Source: three-view drawing plus pictorial views. Frame: mm from the lowest corner of the part. Give positions to 0.01 mm unless a question says otherwise; leave off trailing zeros. Return JSON: item names as keys, results as strings.
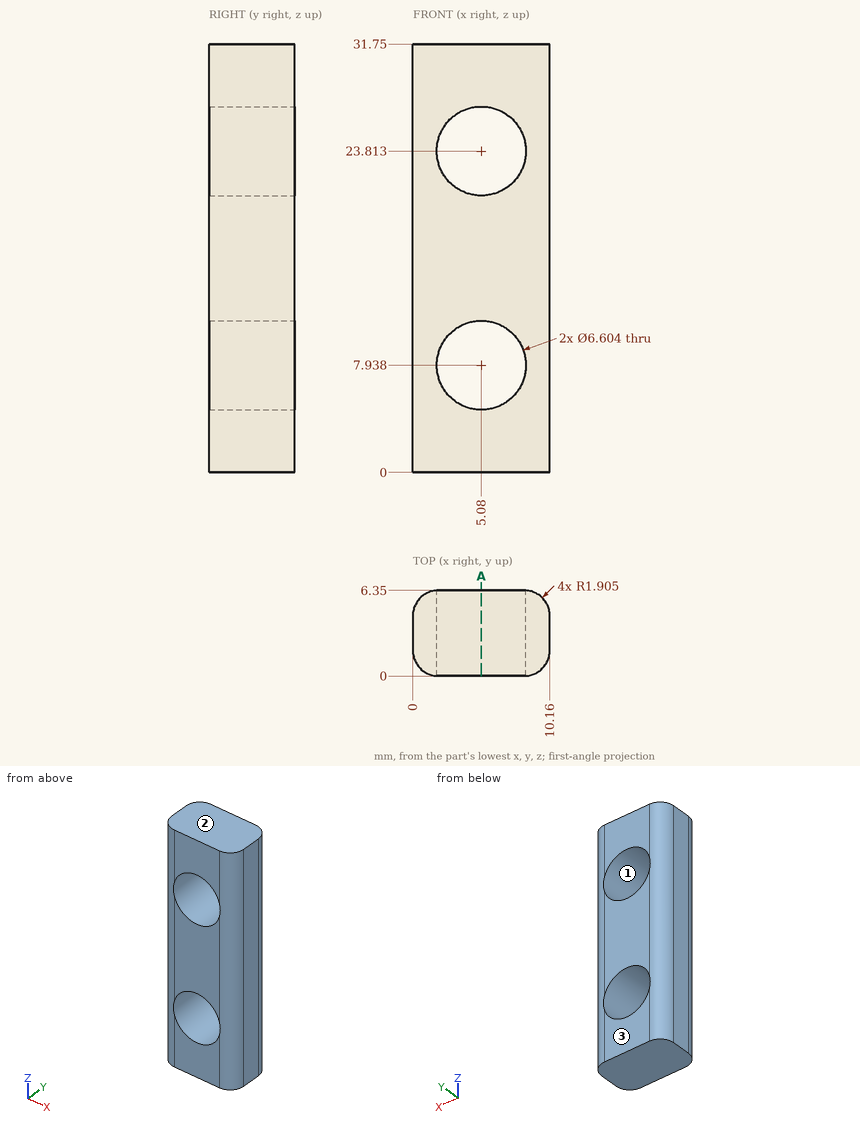
1) Draft query along Z for the marked faces 1, 2 and 3. Return one class per face: released by +Z, released by -Z, zero draft, split by the parting line, or undercut.
Numbers:
{"face 1": "undercut", "face 2": "released by +Z", "face 3": "zero draft"}
2) Cut plane A-A, the plane x = 5.08. Give the number of separate pieces and of enclosed holes in the cut face, then the cut area to 3 significant figures.
Numbers:
{"separate pieces": "3", "enclosed holes": "0", "area": "118 mm²"}
3) Line query: line 1 (X direction, y = 2.5, z = 24.5); line 2 (X direction, y = 6, z = 11.5) (1 decimal); line 3 (X direction, y = 1, z = 22.5). Output: solid intervals per line, ascending. Write a range as [from, to].
Numbers:
{"line 1": "x = [0, 1.85], [8.31, 10.16]", "line 2": "x = [0.8, 9.4]", "line 3": "x = [0.23, 2.05], [8.11, 9.93]"}
4) Contact query for a flat-ended pin moving along its axis: pin 1 Ø1 at (y, z) = (1, 19) entering from -X. Output: stop coordinate, or through.
Numbers:
{"pin 1": "stops at x = 0.04"}
